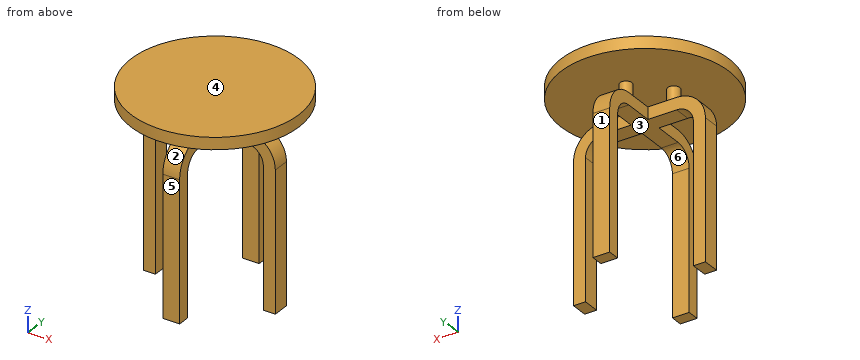
from build123d import *

# Parameters (mm, degrees)
F1_DEPTH = 17.5
F2_COUNT = 2
F2_ANGLE = 90
F4_R     = 175
F5_DEPTH = 25
F6_R     = 12.5
F7_DEPTH = 30
F8_COUNT = 4


with BuildPart() as f1:
    # F0 (on Front) → F1 (new body, symmetric)
    with BuildSketch(Plane.XZ):
        with BuildLine():
            Line((-137.5, 290), (-137.5, 0))
            Line((-137.5, 0), (-112.5, 0))
            Line((-112.5, 0), (-112.5, 290))
            ThreePointArc((-112.5, 290), (-102.248737, 314.748737), (-77.5, 325))
            Line((-77.5, 325), (0, 325))
            Line((0, 325), (77.5, 325))
            ThreePointArc((77.5, 325), (102.248737, 314.748737), (112.5, 290))
            Line((112.5, 290), (112.5, 0))
            Line((112.5, 0), (137.5, 0))
            Line((137.5, 0), (137.5, 290))
            ThreePointArc((137.5, 290), (119.926407, 332.426407), (77.5, 350))
            Line((77.5, 350), (0, 350))
            Line((0, 350), (-77.5, 350))
            ThreePointArc((-77.5, 350), (-119.926407, 332.426407), (-137.5, 290))
        make_face()
    extrude(amount=F1_DEPTH, both=True)

    # F2: F1 ×2 about axis
    f2_axis = Axis((0, 0, 337.5), (0, 0, 1))


with BuildPart() as f1_1:
    add(f1.part)
    for i in range(1, F2_COUNT):
        add(f1.part.rotate(f2_axis, i * F2_ANGLE / (F2_COUNT - 1)))



with BuildPart() as f5:
    # F4 (on offset) → F5 (new body)
    with BuildSketch(Plane.XY.offset(380)):
        Circle(F4_R)
    extrude(amount=F5_DEPTH)


with BuildPart() as f1_2:
    add(f1_1.part)

    add(f5.part)  # F7 merges F5
    # F6 (on face) → F7 (join, through all)
    with BuildSketch(Plane.XY.offset(350)):
        with Locations((-60, 0)):
            Circle(F6_R)
    extrude(amount=F7_DEPTH)

    # F8: F1 ×4 about axis
    f8_axis = Axis((0, 0, 337.5), (0, 0, 1))


with BuildPart() as f1_3:
    add(f1_2.part)
    for i in range(1, F8_COUNT):
        add(f1_2.part.rotate(f8_axis, i * 360 / F8_COUNT))


solid = f1_3.part
Model file for the job. Use its own axes, mm. Face numbers are marked on the shaded views. A direction names the side the tool comes from. Give positions to 0.01 mm unless a question says otherwise; leave off trailing zeros. Write each loop counter-clockwise with the first axis right and the second up, starting at its lowest first coordinate (ties: lowest second). Pieces come first, ordered by that corner, then holes. Notation, with made-up numbers: M 13,0 L 39,0 A12 cw 39,10 Z; hole C -6.75,63 d7. An arc over 180 degrees is marked long. One line per item, written item: value. Start each with the question number.
Q1. Saw through at A-A, the plane x = 0. Write the cut outline in (y, z).
Q2. Saw through at C-C, the plane y = -38.5. Write the cut outline in (x, z).
Q3. Drop flat-ended pins along their axis: pin 1 Ø4 at (y, z) = (116, 283) entering from +X; pin 2 Ø17.5 at (x, z) = (-8, 176) entering from +Y; pin 3 Ø8 at (x, y) = (8.5, -114) entering from -Z; pin 4 Ø4 at (x, z) = (121.5, 331.5) entering from -Y. Give the stop position or say it passes through.
Q4. Two-plate mould, pull along Y, no slides. Class the marked faces 1, 2 and 3: +Y half, -Y half, draft (parallel to the pull), parting line (faces both ways), or undercut.
Q5. 3-axis set-ups, long thin cutter, end or side, ignore diameter. For the marked faces 4, 5 and 6: which of +Z, -Z, +X, -X, +Y, -Y reach the whole face in a straight line?
Q6. Saw through at B-B, the plane z = 138.5. Write the cut outline in (x, y).
Q7. Probe probe 1 along Y at (x, z) = (10, 254.5); probe 2 along Z at (x, y) = (39, 11). List the from-to ranges inside material, lowest first. Write a range as [from, to].
Output values:
1. outline: M -175,380 L -72.5,380 L -72.5,350 L -77.5,350 A60 ccw -137.5,290 L -137.5,0 L -112.5,0 L -112.5,290 A35 cw -77.5,325 L 77.5,325 A35 cw 112.5,290 L 112.5,0 L 137.5,0 L 137.5,290 A60 ccw 77.5,350 L 72.5,350 L 72.5,380 L 175,380 L 175,405 L -175,405 Z; hole M -47.5,350 L 47.5,350 L 47.5,380 L -47.5,380 Z
2. outline: M -170.71,380 L 170.71,380 L 170.71,405 L -170.71,405 Z; M -17.5,325 L 17.5,325 L 17.5,350 L -17.5,350 Z
3. pin 1: stops at x = 17.5
3. pin 2: stops at y = 137.5
3. pin 3: stops at z = 0
3. pin 4: stops at y = -17.5
4. face 1: +Y half
4. face 2: -Y half
4. face 3: undercut
5. face 4: +Z, +X, -X, +Y, -Y
5. face 5: -Z, +X, -X, -Y
5. face 6: -Z, +X, -X
6. outline: M -137.5,-17.5 L -112.5,-17.5 L -112.5,17.5 L -137.5,17.5 Z; M -17.5,-137.5 L 17.5,-137.5 L 17.5,-112.5 L -17.5,-112.5 Z; M -17.5,112.5 L 17.5,112.5 L 17.5,137.5 L -17.5,137.5 Z; M 112.5,-17.5 L 137.5,-17.5 L 137.5,17.5 L 112.5,17.5 Z
7. probe 1: y = [-137.5, -112.5], [112.5, 137.5]
7. probe 2: z = [325, 350], [380, 405]
